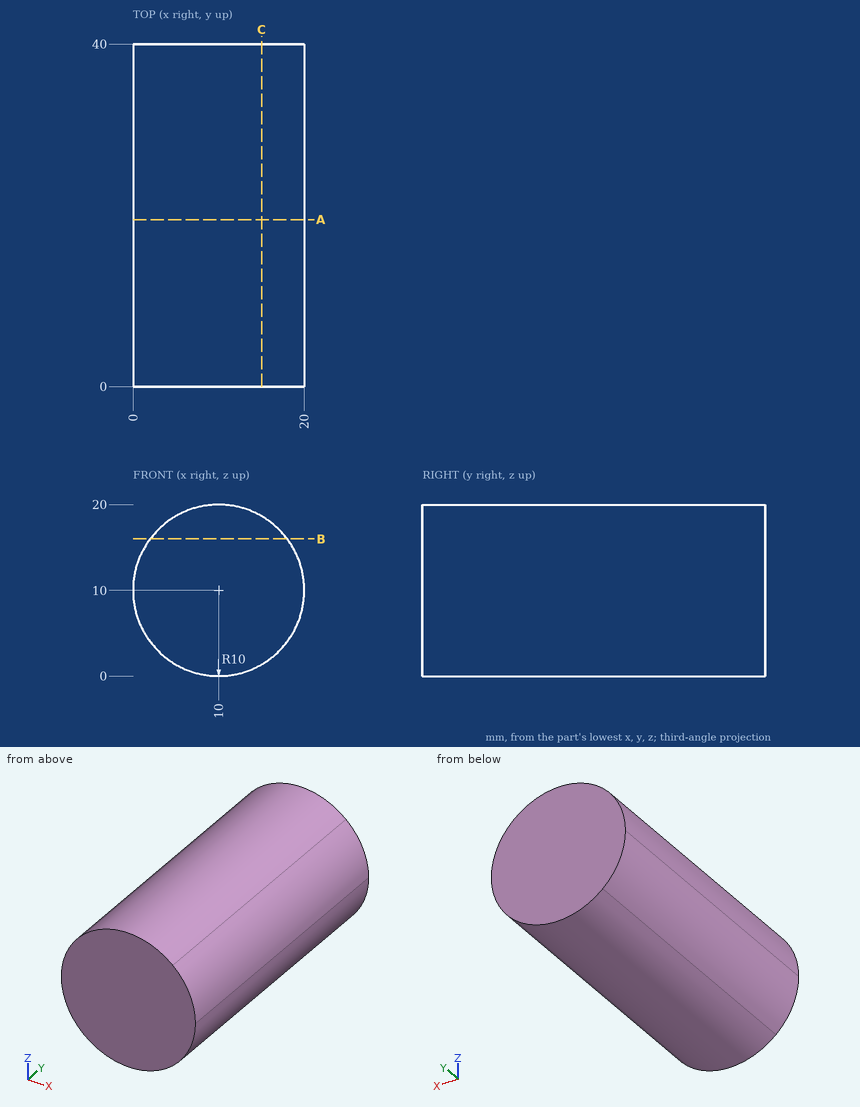
Verification items for this drawing (mm, ordinates from the low corner). Coordinates: 2 decimals unless noted, no trailing zeros. Loops run counter-clockwise (first coordinate to the right, second up) from the corner with the lowest first, then second, coordinate; pieces in that order, holes last. Notation, with made-up numbers: (34, -39) - (53, -39) arc R24 cw to (53, -22) - close; hole circle Ø10 at (3.5, 45). An arc over 180 degrees is marked (long way). One line per item, written item: value. Start each with the question number.
(1) Cross-section at C-C on x = 15. Enter the section's corners in (y, z), plus the area to 3 significant figures.
(2) Depth check by flat-ended pin: P1, Ø1.5, axis at x = 8, y = 27.5, coming from the -Z side. Enter the tip coordinate at first touch or a pass-through.
(3) Material ranges on line 1 (Z direction, x = 9.75, y = 13); line 2 (X direction, y = 29, z = 12); line 3 (Z direction, x = 2, y = 6.5), recorded low to high. Write a range as [from, to].
(4) Cross-section at B-B on z = 16. Enter the section's corners in (x, y), plus the area to 3 significant figures.
(5) Cross-section at A-A on y = 19.5. Enter the section's corners in (x, z).
Results below:
1. outline: (0, 1.34) - (40, 1.34) - (40, 18.66) - (0, 18.66) - close
1. area: 693 mm2
2. P1: stops at z = 0.08
3. line 1: z = [0, 20]
3. line 2: x = [0.2, 19.8]
3. line 3: z = [4, 16]
4. outline: (2, 0) - (18, 0) - (18, 40) - (2, 40) - close
4. area: 640 mm2
5. outline: circle Ø20 at (10, 10)
